from build123d import *

# Parameters (mm, degrees)
CYLINDER025_R             = 3.5
CYLINDER025_DEPTH         = 3
CYLINDER025_PITCH_ANGLE   = 90
CYLINDER024_R             = 2
CYLINDER024_DEPTH         = 9
CYLINDER024_PITCH_ANGLE   = 90
ARRAY021_COUNT            = 2
ARRAY022_Y_COUNT          = 2
ARRAY022_Y_PITCH          = 174
BOX001_W                  = 305
BOX001_H                  = 215
BOX001_DEPTH              = 29
BOX_W                     = 325
BOX_H                     = 235
BOX_DEPTH                 = 29
BOX003_W                  = 288
BOX003_H                  = 198
BOX003_DEPTH              = 6
BOX002_W                  = 325
BOX002_H                  = 235
BOX002_DEPTH              = 6
FUSION017_PLACEMENT_ANGLE = 180


with BuildPart() as case_2_frame_cut002:
    # Cylinder025 → Cylinder025 (new body)
    with BuildSketch(Plane.XY):
        Circle(CYLINDER025_R)
    extrude(amount=CYLINDER025_DEPTH)


with BuildPart() as case_2_frame_cut002_1:
    # Cylinder025 pitch: moved
    add(case_2_frame_cut002.part.rotate(Axis((0, 0, 0), (0, 1, 0)), CYLINDER025_PITCH_ANGLE))


with BuildPart() as case_2_frame_cut002_2:
    # Cylinder025 placement: moved
    add(case_2_frame_cut002_1.part)


with BuildPart() as array022:
    # Cylinder024 → Cylinder024 (new body)
    with BuildSketch(Plane.XY):
        Circle(CYLINDER024_R)
    extrude(amount=CYLINDER024_DEPTH)


with BuildPart() as array022_1:
    # Cylinder024 pitch: moved
    add(array022.part.rotate(Axis((0, 0, 0), (0, 1, 0)), CYLINDER024_PITCH_ANGLE))


with BuildPart() as array022_2:
    # Cylinder024 placement: moved
    add(array022_1.part.moved(Location((3, 0, 0))))

    # Fusion: union CASE_2_frame_cut002
    add(case_2_frame_cut002_2.part)


with BuildPart() as array022_3:
    # Fusion placement: moved
    add(array022_2.part.moved(Location((-163, 87, -14))))

    # Array021: Array022 ×2 about axis
    array021_axis = Axis((0, 87, 0), (0, 0, 1))


with BuildPart() as array022_4:
    add(array022_3.part)
    for i in range(1, ARRAY021_COUNT):
        add(array022_3.part.rotate(array021_axis, i * 360 / ARRAY021_COUNT))

    # Array022 Y: Array022 ×2


with BuildPart() as array022_5:
    add(array022_4.part)
    with Locations(*[(0, -i * ARRAY022_Y_PITCH, 0) for i in range(1, ARRAY022_Y_COUNT)]):
        add(array022_4.part)


with BuildPart() as obj1:
    # Box001 → Box001 (new body)
    with BuildSketch(Plane(origin=(-152.5, -107.5, 0), x_dir=(1, 0, 0), z_dir=(0, 0, 1))):
        with Locations((152.5, 107.5)):
            Rectangle(BOX001_W, BOX001_H)
    extrude(amount=BOX001_DEPTH)


with BuildPart() as case_2_frame_l:
    # Box → Box (new body)
    with BuildSketch(Plane(origin=(-162.5, -117.5, 0), x_dir=(1, 0, 0), z_dir=(0, 0, 1))):
        with Locations((162.5, 117.5)):
            Rectangle(BOX_W, BOX_H)
    extrude(amount=BOX_DEPTH)

    # Cut004: cut obj1
    add(obj1.part, mode=Mode.SUBTRACT)


with BuildPart() as obj2:
    # Box003 → Box003 (new body)
    with BuildSketch(Plane(origin=(-144, -99, 0), x_dir=(1, 0, 0), z_dir=(0, 0, 1))):
        with Locations((144, 99)):
            Rectangle(BOX003_W, BOX003_H)
    extrude(amount=BOX003_DEPTH)


with BuildPart() as case_2_frame_front001:
    # Box002 → Box002 (new body)
    with BuildSketch(Plane(origin=(-162.5, -117.5, 0), x_dir=(1, 0, 0), z_dir=(0, 0, 1))):
        with Locations((162.5, 117.5)):
            Rectangle(BOX002_W, BOX002_H)
    extrude(amount=BOX002_DEPTH)

    # Cut003: cut obj2
    add(obj2.part, mode=Mode.SUBTRACT)


with BuildPart() as case_2_frame_front001_1:
    # Cut003 placement: moved
    add(case_2_frame_front001.part.moved(Location((0, 0, -6))))

    # Fusion017: union CASE_2_frame_l
    add(case_2_frame_l.part)


with BuildPart() as case_2_frame_front001_2:
    # Fusion017 placement: moved
    add(case_2_frame_front001_1.part.rotate(Axis((0, 0, 0), (0, 1, 0)), FUSION017_PLACEMENT_ANGLE))

    # Cut: cut Array022
    add(array022_5.part, mode=Mode.SUBTRACT)


solid = case_2_frame_front001_2.part
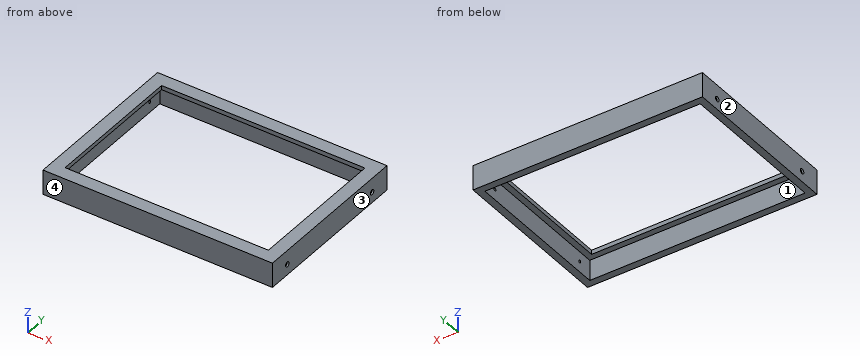
The listing builds one solid part. Answer for the finished solid, in the listing's coordinates (mm). Face numbers are marked on the shaded views. Give positions to 0.01 mm unless a question says otherwise; leave off trailing zeros. Write each loop counter-clockwise with the first axis right and the second up, starting at its lowest first coordinate (ties: lowest second). Pieces come first, ordered by that corner, then holes. Notation, with made-up numbers: (13, 58.5) -> (44, 58.5) arc R24 cw to (44, 73.5) -> close; hole circle Ø2 at (85.5, -34). An arc over 180 degrees is marked (long way). One line per question, with ' | ' between items. Start each with the question number.
1. Section B-B (z = -25) is taken. Determine the outline of the cut face in (x, y).
2. For a pull along X with two mould halves and no side action, classify the marked faces 1, 2, 3 and 4 as pulls with the +X half, pulls with the -X half, needs draft (parallel to the pull), parting line crosses it, or undercut.
3. Section A-A (x = 50) is taken. Determine the outline of the cut face in (y, z), plus the area to 3 significant figures.
4. Given pin 1 Ø5.5 at (y, z) = (-87, -14) entering from -X, flat-ended and moving along its own axis, determine where the tip first touches the part or whether it passes through.
5. Section C-C (y = -43) is taken. Determine the outline of the cut face in (x, z), plus the area to 3 significant figures.
6. Find the intervals of material crossed by probe 1 along Y at (x, z) = (161.7, -14); probe 2 along X at (y, z) = (57, -11); probe 3 along Y at (x, z) = (154.75, -14), in increasing order.
Response values:
1) outline: (-162.5, -117.5) -> (162.5, -117.5) -> (162.5, 117.5) -> (-162.5, 117.5) -> close; hole (-152.5, -107.5) -> (152.5, -107.5) -> (152.5, 107.5) -> (-152.5, 107.5) -> close
2) face 1: undercut | face 2: pulls with the -X half | face 3: pulls with the +X half | face 4: needs draft
3) outline: (-117.5, -29) -> (-107.5, -29) -> (-107.5, 0) -> (-99, 0) -> (-99, 6) -> (-117.5, 6) -> close; (99, 0) -> (107.5, 0) -> (107.5, -29) -> (117.5, -29) -> (117.5, 6) -> (99, 6) -> close | area: 802 mm2
4) pin 1: x = -160
5) outline: (-162.5, -29) -> (-152.5, -29) -> (-152.5, 0) -> (-144, 0) -> (-144, 6) -> (-162.5, 6) -> close; (144, 0) -> (152.5, 0) -> (152.5, -29) -> (162.5, -29) -> (162.5, 6) -> (144, 6) -> close | area: 802 mm2
6) probe 1: -117.5 to -90.5, -83.5 to 83.5, 90.5 to 117.5 | probe 2: -162.5 to -152.5, 152.5 to 162.5 | probe 3: -117.5 to -89, -85 to 85, 89 to 117.5
